Model file for the job. Use its own axes, mm. A direction names the side the tool comes from. Round coordinates to 2 decimals unless told otherwise and drop trailing zeros. Loops run counter-clockwise (first coordinate to the right, second up) from the corner with the lowest first, then second, coordinate; pieces in that order, holes last. Notation, with made-up numbers: M -31,49.5 L 18,49.5 A4 ccw 18,55.5 Z; hole C -21,84 d4. An arc over 180 degrees is marked long. Use a Markdown table: item, result. Add a question column.
Item 1: Saw through at A-A on y = 39.5. Write the cut outline in (x, z).
Item 2: Tool access for faces 4 (the cylindrical face through (110.885, 55.261, -0.789)), 5 (the flat face through (128, 45, -2)): list every direction of +Z, -Z, +X, -X, +Y, -Y with a clear straight run to the whole face (end or side of a thin tool).
Item 3: Saw through at B-B on x = 113.5. Write the cut outline in (y, z), then the cut area to 3 significant figures.
Item 4: Pin check, flat tips, straight feed: P1, Ø2.5, axis at x = 124.89, y = 55.33, coming from the -Z side; P2, Ø2, axis at x = 109, z = 0.5, coming from the +Y side. Stop position of each tip, or through.
Item 5: Two-plate mould, pull along X, no slides. Class faces 1 (the cylindrical face through (110.885, 35.261, -0.789)), 2 (the cylindrical face through (112.763, 40.176, 0.986)), 3 (the flat face through (113, 34, 0)): +X half, -X half, draft (parallel to the pull), parting line (faces both ways), or undercut.
Item 6: Saw through at C-C on x = 108.5. Write the cut outline in (y, z), then the cut area to 3 significant figures.
Item 7: Wall check: L1, parallel to Y at x = 113.5, z = 1.6; L2, parallel to Z at x = 111.5, y = 21; L3, parallel to X at y = 55, z = 1.55. Give the ranges that are in metal, low to high. Write a range as from..to.
Item 8: Saw through at D-D on y = 44.51. Write the cut outline in (x, z), then the cut area to 3 significant figures.
```python
from build123d import *

# Parameters (mm, degrees)
SKETCH_R     = 24.107232
SKETCH_R_2   = 1
PAD_DEPTH    = 2
SKETCH001_R  = 2.5
PAD001_DEPTH = 4
CHAMFER_SIZE = 0.4


with BuildPart() as part:
    # Sketch → Pad (new body)
    with BuildSketch(Plane.XY):
        with Locations((113.5, 39.5)):
            Circle(SKETCH_R)
        with Locations((124.893001, 55.325597)):
            Circle(SKETCH_R_2, mode=Mode.SUBTRACT)
        with Locations((94.09813, 41.45383)):
            Circle(SKETCH_R_2, mode=Mode.SUBTRACT)
        with Locations((121.508868, 21.720573)):
            Circle(SKETCH_R_2, mode=Mode.SUBTRACT)
        with Locations((113.5, 39.5)):
            Circle(SKETCH_R_2, mode=Mode.SUBTRACT)
    extrude(amount=PAD_DEPTH)

    # Sketch001 (on Face7 of Pad) → Pad001 (join)
    with BuildSketch(Plane.XY.offset(2)):
        with Locations((108.5, 34.51)):
            Circle(SKETCH001_R)
        with Locations((108.5, 54.51)):
            Circle(SKETCH001_R)
        with Locations((128.5, 44.51)):
            Circle(SKETCH001_R)
    extrude(amount=-PAD001_DEPTH)

    # Chamfer
    chamfer_edges = [part.edges().sort_by_distance(p)[0] for p in [
        (106, 34.51, -2),
        (106, 54.51, -2),
        (126, 44.51, -2),
    ]]
    chamfer(chamfer_edges, length=CHAMFER_SIZE)


solid = part.part
```
Entries:
| question | item | result |
|---|---|---|
| 1 | outline | M 89.39,0 L 112.5,0 L 112.5,2 L 89.39,2 Z; M 114.5,0 L 137.61,0 L 137.61,2 L 114.5,2 Z |
| 2 | face 4 | -Z |
| 2 | face 5 | -Z, +X, -X, +Y, -Y |
| 3 | outline | M 15.39,0 L 38.5,0 L 38.5,2 L 15.39,2 Z; M 40.5,0 L 63.61,0 L 63.61,2 L 40.5,2 Z |
| 3 | area | 92.4 mm2 |
| 4 | P1 | z = 0 |
| 4 | P2 | y = 63.35 |
| 5 | face 1 | parting line |
| 5 | face 2 | undercut |
| 5 | face 3 | draft |
| 6 | outline | M 15.92,0 L 32.01,0 L 32.01,-1.6 L 32.41,-2 L 36.61,-2 L 37.01,-1.6 L 37.01,0 L 52.01,0 L 52.01,-1.6 L 52.41,-2 L 56.61,-2 L 57.01,-1.6 L 57.01,0 L 63.08,0 L 63.08,2 L 15.92,2 Z |
| 6 | area | 114 mm2 |
| 7 | L1 | 15.39..38.5, 40.5..63.61 |
| 7 | L2 | 0..2 |
| 7 | L3 | 95.04..123.95, 125.84..131.96 |
| 8 | outline | M 89.92,0 L 126,0 L 126,-1.6 L 126.4,-2 L 130.6,-2 L 131,-1.6 L 131,0 L 137.08,0 L 137.08,2 L 89.92,2 Z |
| 8 | area | 104 mm2 |
